Could you check a few things on this model? Use its own coordinates, in mm. Face numbers are marked on the shaded views. A direction names the side the tool comes from. Round coordinates to 2 decimals unless told otherwise and drop trailing zeros. Write each loop counter-clockwise with the first axis right and the second up, starting at its lowest first coordinate (ties: lowest second). Pieces come first, ordered by that corner, then holes. Notation, with made-up numbers: (72, 35.5) -> (125, 35.5) arc R11 ccw to (125, 42.5) -> close; hole circle Ø8 at (2.5, -33). An arc over 180 degrees is marked (long way). One line per question, with ' | ' between items. Start each with the question number.
1. For pin 1 Ø3 at (x, z) = (-1.5, 7) entering from -Y; pin 2 Ø8 at (x, y) = (8.5, 5.5) entering from -Z; pin 3 Ø8 at (x, z) = (4, 5.5) entering from -Y; pin 4 Ø4 at (x, y) = (10, 7) entering from -Z, each with a flat end and sliding along its axis, tell me the tip position at first contact or that it passes through.
2. If I drill on line 1 along Z through (x, y) = (0.5, -8.5); line 2 along Y through (x, z) = (-7, 2.75); line 3 along X through (y, z) = (7.5, 1.75), over which ranges is the centre line in solid material (lowest first)? Write a range as [from, to].
3. Imagine slicing it at C-C, the plane z = 8.5. List the corners of the cut face in (x, y) for me.
4. Imagine slicing it at D-D, the plane z = 1.5. List the corners of the cut face in (x, y) for me, and give its area (3 significant figures).
5. For the marked faces 1 and 2, which set-ups out of +Z, -Z, +X, -X, +Y, -Y let a thin tool reach every point of the face, with its end or its side?
6. Imagine slicing it at A-A, the plane y = 0. List the corners of the cut face in (x, z) for me (3 decimals).
from build123d import *

# Parameters (mm, degrees)
SKETCH1_R           = 12.7
BOSS_EXTRUDE1_DEPTH = 12.7
SKETCH4_R           = 7.62
BOSS_EXTRUDE2_DEPTH = 2.54


with BuildPart() as part:
    # Sketch1 → Boss-Extrude1 (new body)
    with BuildSketch(Plane.XY):
        Circle(SKETCH1_R)
    extrude(amount=BOSS_EXTRUDE1_DEPTH)

    # Sketch2 → Cut-Revolve1 (revolve, cut)
    with BuildSketch(Plane(origin=(0, 0, 0), x_dir=(0, 0, -1), z_dir=(1, 0, 0)), mode=Mode.PRIVATE) as cut_revolve1_sk:
        with BuildLine():
            Line((-12.065, 12.7), (-0.635, 12.7))
            ThreePointArc((-0.635, 12.7), (-6.35, 6.985), (-12.065, 12.7))
        make_face()
    revolve(cut_revolve1_sk.sketch.rotate(Axis((0, 0, 6.35), (0, 0, 1)), 90), axis=Axis((0, 0, 6.35), (0, 0, 1)), mode=Mode.SUBTRACT)

    # Sketch4 → Boss-Extrude2 (add)
    with BuildSketch(Plane(origin=(0, 0, 0), x_dir=(-1, 0, 0), z_dir=(0, 0, -1))):
        Circle(SKETCH4_R)
    extrude(amount=BOSS_EXTRUDE2_DEPTH)


solid = part.part
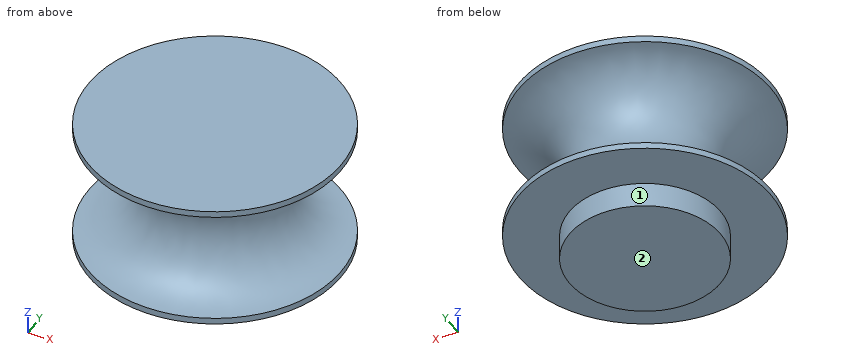
Geometry results:
1) pin 1: stops at y = -7.3 | pin 2: stops at z = -2.54 | pin 3: stops at y = -9 | pin 4: stops at z = 0
2) line 1: z = [0, 2.46], [10.24, 12.7] | line 2: y = [-4.39, 4.39] | line 3: x = [-5.51, 5.51]
3) outline: circle Ø14.81 at (0, 0)
4) outline: circle Ø19.35 at (0, 0) | area: 294 mm2
5) face 1: -Z | face 2: -Z, +X, -X, +Y, -Y
6) outline: (-12.7, 0) -> (-7.62, 0) -> (-7.62, -2.54) -> (7.62, -2.54) -> (7.62, 0) -> (12.7, 0) -> (12.7, 0.635) arc R5.715 cw to (12.7, 12.065) -> (12.7, 12.7) -> (-12.7, 12.7) -> (-12.7, 12.065) arc R5.715 cw to (-12.7, 0.635) -> close
